The model under review builds one solid part; all positions refer to its coordinate system, in mm. A direction names the side the tool comes from. Round coordinates to 2 decimals unless told otherwise and drop trailing zeros. Loops run counter-clockwise (first coordinate to the right, second up) from the corner with the lowest first, then second, coordinate; pieces in that order, holes last. Notation, with made-up numbers: (-26.5, 68) -> (21.5, 68) arc R22 cw to (21.5, 87) -> close; hole circle Ø8 at (69.5, 27). An arc over 180 degrees is marked (long way). Write each question's results on one line, items separated by ' | '. Start each with the question number.
Item 1: We need section D-D (z = -20). Give the number of separate pieces and of enclosed holes in the cut face, and give its area (3 significant figures).
Item 2: Clearance check with flat-ended pins moving along their axes: pin 1 Ø10 at (y, z) = (60, 20) entering from -X; pin 2 Ø1.3 at (x, z) = (-0.5, -21) entering from -Y; pin 3 Ø0.8 at (x, z) = (-1, 21) entering from +Y; pin 4 Ø5 at (y, z) = (60, -20) entering from -X. State where each tip first meets the part, or that it passes through.
Item 3: For L1, parallel to X at y = 4.75, z = -20; L2, parallel to Z at x = 10.5, y = 11, list the stretches that pass through material, from the lowest coordinate up. Write a range as from..to.
Item 4: Tool access review of faces 1 (the cylindrical face through (3.3, 44.25, -19.91)), 2 (the flat face through (4, -1, 16)), 3 (the flat face through (4, -1, -24)): name each direction out of +Z, -Z, +X, -X, +Y, -Y from which nothing blocks a thin tool from reaching the whole face with its end or side.
Item 5: We need section C-C (y = 16). Give the boundary of the cut face in (x, z), and give its area (3 significant figures).
Item 6: We need section A-A (y = 60). Give the boundary of the cut face in (x, z), and give its area (4 significant figures).
Item 7: Mouldability with a two-part tool opening along Z and no side actions: class faces 4 (the flat face through (-1, 73, -24)), 5 (the flat face through (-2.5, 73, -20)), 6 (the flat face through (-1, 4, 16)) as pulls with the +Z half, pulls with the -Z half, needs draft (parallel to the pull), parting line crosses it, or undercut.
Item 8: We need section B-B (x = 16.5). Give the boundary of the cut face in (y, z), and give its area (3 significant figures).
from build123d import *

# Parameters (mm, degrees)
EXTRUDE_1_DEPTH     = 39
EXTRUDE_2_DEPTH     = 4
SKETCH_3_R          = 4.25
CUT_EXTRUDE_1_DEPTH = 7.5
SKETCH_4_W          = 3
SKETCH_4_H          = 8
EXTRUDE_3_DEPTH     = 2.5


with BuildPart() as part:
    # Эскиз1 → Бобышка-Вытянуть1 (new body, symmetric)
    with BuildSketch(Plane.XY):
        Polygon((0, 78), (0, 0), (78, 0), (78, 6.5), (6.5, 6.5), (6.5, 78), align=None)
    extrude(amount=EXTRUDE_1_DEPTH, both=True)

    # Эскиз2 → Бобышка-Вытянуть2 (add)
    with BuildSketch(Plane.XY.offset(39)):
        with BuildLine():
            Line((78, 6.5), (6.5, 6.5))
            Line((6.5, 6.5), (6.5, 78))
            Line((6.5, 78), (9.5, 78))
            ThreePointArc((9.5, 78), (11.621320344, 77.121320344), (12.5, 75))
            Line((12.5, 75), (12.5, 73))
            Line((12.5, 73), (73, 12.5))
            Line((73, 12.5), (75, 12.5))
            ThreePointArc((75, 12.5), (77.121320344, 11.621320344), (78, 9.5))
            Line((78, 9.5), (78, 6.5))
        make_face()
    extrude_2 = extrude(amount=-EXTRUDE_2_DEPTH)

    # Зеркальное отражение2: Бобышка-Вытянуть2 across plane
    add(extrude_2.mirror(Plane.XY))

    # Эскиз3 → Вырез-Вытянуть1 (cut, through all)
    with BuildSketch(Plane(origin=(0, 6.5, 0), x_dir=(1, 0, 0), z_dir=(0, 1, 0))):
        with Locations(Location((60, -20, 0), (0, 0, 270))):  # turned: the seam where the file's is
            Circle(SKETCH_3_R)
        with Locations(Location((60, 20, 0), (0, 0, 90))):  # turned: the seam where the file's is
            Circle(SKETCH_3_R)
        with BuildLine():
            Line((23, -15.75), (40, -15.75))
            ThreePointArc((40, -15.75), (44.25, -20), (40, -24.25))
            Line((40, -24.25), (23, -24.25))
            ThreePointArc((23, -24.25), (18.75, -20), (23, -15.75))
        make_face()
        with BuildLine():
            Line((23, 15.75), (40, 15.75))
            ThreePointArc((40, 15.75), (44.25, 20), (40, 24.25))
            Line((40, 24.25), (23, 24.25))
            ThreePointArc((23, 24.25), (18.75, 20), (23, 15.75))
        make_face()
    cut_extrude_1 = extrude(amount=-CUT_EXTRUDE_1_DEPTH, mode=Mode.SUBTRACT)

    # Эскиз4 → Бобышка-Вытянуть3 (add)
    with BuildSketch(Plane.XZ):
        with Locations((4.5, -20)):
            Rectangle(SKETCH_4_W, SKETCH_4_H)
        with Locations((73.5, -20)):
            Rectangle(SKETCH_4_W, SKETCH_4_H)
        with Locations((73.5, 20)):
            Rectangle(SKETCH_4_W, SKETCH_4_H)
        with Locations((4.5, 20)):
            Rectangle(SKETCH_4_W, SKETCH_4_H)
    extrude_3 = extrude(amount=EXTRUDE_3_DEPTH)

    # Зеркальное отражение3: Вырез-Вытянуть1, Бобышка-Вытянуть3 across plane
    add(cut_extrude_1.mirror(Plane(origin=(0, 0, 0), x_dir=(0, 0, 1), z_dir=(-0.707106781, 0.707106781, 0))), mode=Mode.SUBTRACT)
    add(extrude_3.mirror(Plane(origin=(0, 0, 0), x_dir=(0, 0, 1), z_dir=(-0.707106781, 0.707106781, 0))))


solid = part.part
Here are the results:
1) separate pieces: 5 | enclosed holes: 0 | area: 560 mm2
2) pin 1: stops at x = 0 | pin 2: stops at y = 0 | pin 3: stops at y = 75 | pin 4: passes through
3) L1: x = -2.5..18.75, 44.25..55.75, 64.25..78 | L2: z = -39..-35, 35..39
4) face 1: +X, -X | face 2: +X, -X, -Y | face 3: -Z, +X, -X, -Y
5) outline: (0, -39) -> (69.5, -39) -> (69.5, -35) -> (6.5, -35) -> (6.5, 35) -> (69.5, 35) -> (69.5, 39) -> (0, 39) -> close | area: 1,010 mm2
6) outline: (0, -39) -> (25.5, -39) -> (25.5, -35) -> (6.5, -35) -> (6.5, -24.25) -> (0, -24.25) -> close; (0, -15.75) -> (6.5, -15.75) -> (6.5, 15.75) -> (0, 15.75) -> close; (0, 24.25) -> (6.5, 24.25) -> (6.5, 35) -> (25.5, 35) -> (25.5, 39) -> (0, 39) -> close | area: 548.5 mm2
7) face 4: pulls with the -Z half | face 5: needs draft | face 6: undercut
8) outline: (0, -39) -> (69, -39) -> (69, -35) -> (6.5, -35) -> (6.5, 35) -> (69, 35) -> (69, 39) -> (0, 39) -> close | area: 1,010 mm2
